```python
from build123d import *

# Parameters (mm, degrees)
F0_W     = 250
F0_H     = 116
F1_DEPTH = 6
F2_W     = 6
F2_H     = 10
F2_H_2   = 20
F2_W_2   = 26
F2_R     = 1.6
F2_W_3   = 52
F2_H_3   = 16
F3_DEPTH = 6.001
F4_R     = 3
F5_R     = 10
F6_R     = 7.99999
F7_R     = 1.6
F7_W     = 6
F7_H     = 10
F8_DEPTH = 6.0010001


# Not quite as in the source:
# - a fillet or chamfer is up to 0.001 mm smaller than in the source, because OpenCascade refuses the exact size


with BuildPart() as f1:
    # F0 (on Top) → F1 (new body)
    with BuildSketch(Plane.XY):
        Rectangle(F0_W, F0_H)
    extrude(amount=F1_DEPTH)

    # F2 (on face) → F3 (cut, through all)
    with BuildSketch(Plane.XY.offset(6)):
        with Locations((-87, -40)):
            Rectangle(F2_W, F2_H)
        with Locations((-87, 10)):
            Rectangle(F2_W, F2_H)
        with Locations((87, -40)):
            Rectangle(F2_W, F2_H)
        with Locations((87, 10)):
            Rectangle(F2_W, F2_H)
        with Locations((-87, -15)):
            Rectangle(F2_W, F2_H_2)
        with Locations((87, -15)):
            Rectangle(F2_W, F2_H_2)
        with Locations((0, -53)):
            Rectangle(F2_W_2, F2_H)
        with Locations((-87, -30)):
            Circle(F2_R)
        with Locations((-87, 0)):
            Circle(F2_R)
        with Locations((87, -30)):
            Circle(F2_R)
        with Locations((87, 0)):
            Circle(F2_R)
        with BuildLine():
            Line((37, -58), (63, -58))
            Line((63, -58), (63, -52))
            ThreePointArc((63, -52), (50, -39), (37, -52))
            Line((37, -52), (37, -58))
        make_face()
        with Locations((-50, -50)):
            Rectangle(F2_W_3, F2_H_3)
    extrude(amount=-F3_DEPTH, mode=Mode.SUBTRACT)

    # F4
    f4_edges = [f1.edges().sort_by_distance(p)[0] for p in [
        (-13, -48, 3),
        (13, -48, 3),
        (-13, -58, 3),
        (13, -58, 3),
    ]]
    fillet(f4_edges, radius=F4_R)

    # F5
    f5_edges = [f1.edges().sort_by_distance(p)[0] for p in [
        (-125, -58, 3),
        (125, -58, 3),
        (125, 58, 3),
        (-125, 58, 3),
    ]]
    fillet(f5_edges, radius=F5_R)

    # F6 (radius 8 in the source; OpenCascade refuses exactly that, so slightly less here)
    f6_edges = [f1.edges().sort_by_distance(p)[0] for p in [
        (37, -58, 3),
        (63, -58, 3),
        (-24, -58, 3),
        (-24, -42, 3),
        (-76, -42, 3),
        (-76, -58, 3),
    ]]
    fillet(f6_edges, radius=F6_R)

    # F7 (on face) → F8 (cut, through all)
    with BuildSketch(Plane.XY.offset(6)):
        with Locations((-50, 20)):
            Circle(F7_R)
        with Locations((-50, 30)):
            Rectangle(F7_W, F7_H)
        with Locations((50, 30)):
            Rectangle(F7_W, F7_H)
        with Locations((50, 20)):
            Circle(F7_R)
    extrude(amount=-F8_DEPTH, mode=Mode.SUBTRACT)


solid = f1.part
```
For this review, take the finished solid that the model builds, in its own axes (mm). A direction names the side the tool comes from. Give positions to 0.01 mm unless a question says otherwise; leave off trailing zeros. One line per item, written item: value. Start each with the question number.
Q1. Clearance check with flat-ended pins moving along their axes: pin 1 Ø1.9 at (x, y) = (-50, 20) entering from +Z; pin 2 Ø3 at (y, z) = (-53, 4.5) entering from -X; pin 3 Ø2 at (x, z) = (8, 2) entering from -Y. State where each tip first meets the part, or that it passes through.
Q2. Machinability: for faces 1 (the face through (-90, 10, 3)), 2 (the face through (-73.719, -44.406, 2.958)), 3 (the face through (-125, -1, 3)), which of the approach directions +Z, -Z, +X, -X, +Y, -Y give a long, thin tool a straight path to every point of the face, cutting with its end or side? Answer none if there is none.
Q3. For L1, parallel to Y at x = -50, z = 1.7; L2, parallel to X at y = -20, z = 1.75; L3, parallel to Y at x = 50, z = 3.25, list the stretches that pass through material, from the lowest coordinate up.
Q4. Draft analysis for pull direction X (two halves, no side actions). For faces 4 (the face through (-2, 58, 3)), 5 (the face through (-121.99, 55.15, 3.04)), 6 (the face through (87, -45, 3)), state which applies: released by +X, released by -X, zero draft, split by the parting line, or undercut.
Q5. Add section A-A (z = 1.25). Count the separate pieces of the cut face and the enclosed holes in it, and give its area (3 significant figures).
Reply:
1. pin 1: through
1. pin 2: x = -124.37
1. pin 3: y = -48
2. face 1: +Z, -Z
2. face 2: +Z, -Z, -Y
2. face 3: +Z, -Z, -X, +Y, -Y
3. L1: -42 to 18.4, 21.6 to 25, 35 to 58
3. L2: -125 to -90, -84 to 84, 90 to 125
3. L3: -39 to 18.4, 21.6 to 25, 35 to 58
4. face 4: zero draft
4. face 5: released by -X
4. face 6: undercut
5. separate pieces: 1
5. enclosed holes: 14
5. area: 26,700 mm²
